from build123d import *

# Parameters (mm, degrees)
F0_W     = 350
F0_H     = 150
F0_R     = 1.64084
F0_W_2   = 14.666667
F0_H_2   = 3.175
F0_W_3   = 12.7
F0_W_4   = 3.175
F0_H_3   = 5.08
F0_H_4   = 3.215846
F0_R_2   = 3.302
F1_DEPTH = 3.175


with BuildPart() as f1:
    # F0 (on Front) → F1 (new body)
    with BuildSketch(Plane.XZ):
        Rectangle(F0_W, F0_H)
        with Locations((-125.9747, -52.45)):
            Circle(F0_R, mode=Mode.SUBTRACT)
        with Locations((-99.0253, -52.45)):
            Circle(F0_R, mode=Mode.SUBTRACT)
        with Locations((-76.366667, -69.285)):
            Rectangle(F0_W_2, F0_H_2, mode=Mode.SUBTRACT)
        with Locations((-47.033333, -69.285)):
            Rectangle(F0_W_2, F0_H_2, mode=Mode.SUBTRACT)
        with Locations((-130.175, -25.590497)):
            Rectangle(F0_W_3, F0_H_2, mode=Mode.SUBTRACT)
        with Locations((-104.775, -25.590497)):
            Rectangle(F0_W_3, F0_H_2, mode=Mode.SUBTRACT)
        with Locations((-157.1625, -10.032997)):
            Rectangle(F0_W_4, F0_H_3, mode=Mode.SUBTRACT)
        with Locations((-79.375, -25.590497)):
            Rectangle(F0_W_3, F0_H_2, mode=Mode.SUBTRACT)
        with Locations((-53.975, -25.590497)):
            Rectangle(F0_W_3, F0_H_2, mode=Mode.SUBTRACT)
        with Locations((-28.575, -25.590497)):
            Rectangle(F0_W_3, F0_H_2, mode=Mode.SUBTRACT)
        with Locations((-1.5875, -10.032997)):
            Rectangle(F0_W_4, F0_H_3, mode=Mode.SUBTRACT)
        with Locations((99.0253, -52.45)):
            Circle(F0_R, mode=Mode.SUBTRACT)
        with Locations((125.9747, -52.45)):
            Circle(F0_R, mode=Mode.SUBTRACT)
        with Locations((86.7, -12.720423)):
            Rectangle(F0_W_3, F0_H_4, mode=Mode.SUBTRACT)
        with Locations((112.1, -12.720423)):
            Rectangle(F0_W_3, F0_H_4, mode=Mode.SUBTRACT)
        with Locations((-157.1625, 0.127003)):
            Rectangle(F0_W_4, F0_H_3, mode=Mode.SUBTRACT)
        with Locations((-157.1625, 10.287003)):
            Rectangle(F0_W_4, F0_H_3, mode=Mode.SUBTRACT)
        with Locations((-130.175, 25.844503)):
            Rectangle(F0_W_3, F0_H_2, mode=Mode.SUBTRACT)
        with Locations((-104.775, 25.844503)):
            Rectangle(F0_W_3, F0_H_2, mode=Mode.SUBTRACT)
        with Locations((-1.5875, 0.127003)):
            Rectangle(F0_W_4, F0_H_3, mode=Mode.SUBTRACT)
        with Locations((-1.5875, 10.287003)):
            Rectangle(F0_W_4, F0_H_3, mode=Mode.SUBTRACT)
        with Locations((-79.375, 25.844503)):
            Rectangle(F0_W_3, F0_H_2, mode=Mode.SUBTRACT)
        with Locations((-53.975, 25.844503)):
            Rectangle(F0_W_3, F0_H_2, mode=Mode.SUBTRACT)
        with Locations((-28.575, 25.844503)):
            Rectangle(F0_W_3, F0_H_2, mode=Mode.SUBTRACT)
        with Locations((-125.9747, 52.45)):
            Circle(F0_R, mode=Mode.SUBTRACT)
        with Locations((-99.0253, 52.45)):
            Circle(F0_R, mode=Mode.SUBTRACT)
        with Locations((-76.366667, 69.285)):
            Rectangle(F0_W_2, F0_H_2, mode=Mode.SUBTRACT)
        with Locations((-47.033333, 69.285)):
            Rectangle(F0_W_2, F0_H_2, mode=Mode.SUBTRACT)
        Polygon((131.55, 7.9375), (131.55, -7.9375), (93.45, -7.9375), (55.35, -7.9375), (42.65, -7.9375), (42.65, 7.9375), (55.35, 7.9375), (93.45, 7.9375), align=None, mode=Mode.SUBTRACT)
        with Locations((152.14, 0)):
            Circle(F0_R_2, mode=Mode.SUBTRACT)
        with Locations((99.0253, 52.45)):
            Circle(F0_R, mode=Mode.SUBTRACT)
        with Locations((125.9747, 52.45)):
            Circle(F0_R, mode=Mode.SUBTRACT)
    extrude(amount=F1_DEPTH)


solid = f1.part
Input: part model. Units: mm. Frame: model coordinates. Coordinates: 2 decimals unless noted, no trailing zeros. Loops run counter-clockwise (first coordinate to the right, second up) from the corner with the lowest first, then second, coordinate; pieces in that order, holes last. Notation, with made-up numbers: (72, 64) -> (129, 64) arc R23 cw to (129, 90) -> close; hole circle Ø1 at (-25, 59). An arc over 180 degrees is marked (long way). Write each question's results on one line, items separated by ' | '. Start each with the question number.
Q1. Section B-B, the plane x = 109.5. Return the cut outline in (y, z) (1 decimal), plus the area to 3 significant figures.
Q2. Section D-D, the plane y = -1.9. State how many separate pieces and enclosed holes the cut face has, plus the area to 3 significant figures.
Q3. Section C-C, the plane x = 68.5. Return the cut outline in (y, z) (1 decimal).
Q4. Section A-A, the plane x = 152.14. Return the cut outline in (y, z) (3 decimals), plus the area to 3 significant figures.
Q5. Pull-direction query (X, two-part tool) for faces 1 (the flat face through (-2, -3.175, -16)), 2 (the cylindrical face through (148.84, -1.57, 0.15)); classes: released by +X, released by -X, zero draft, split by the parting line, or undercut.
Q6. Ray query, line 1 (X direction, y = -1.9, z = 68); line 2 (Z direction, x = 113.5, y = -0.55); line 3 (X direction, y = -1.9, z = -8.5) (3 decimals). Return the intervals inside material, ascending. Write a range as from..to.
Found:
1) outline: (-3.2, -75) -> (0, -75) -> (0, -14.3) -> (-3.2, -14.3) -> close; (-3.2, -11.1) -> (0, -11.1) -> (0, -7.9) -> (-3.2, -7.9) -> close; (-3.2, 7.9) -> (0, 7.9) -> (0, 75) -> (-3.2, 75) -> close | area: 416 mm2
2) separate pieces: 1 | enclosed holes: 32 | area: 50,200 mm2
3) outline: (-3.2, -75) -> (0, -75) -> (0, -7.9) -> (-3.2, -7.9) -> close; (-3.2, 7.9) -> (0, 7.9) -> (0, 75) -> (-3.2, 75) -> close
4) outline: (-3.175, -75) -> (0, -75) -> (0, -3.302) -> (-3.175, -3.302) -> close; (-3.175, 3.302) -> (0, 3.302) -> (0, 75) -> (-3.175, 75) -> close | area: 455 mm2
5) face 1: zero draft | face 2: undercut
6) line 1: -175..-83.7, -69.03..-54.37, -39.7..175 | line 2: -75..-14.33, -11.11..-7.94, 7.94..75 | line 3: -175..-158.75, -155.575..-3.175, 0..175
